Verification items for the finished model (mm, model axes). Face numbers are marked on the shaded views. A direction names the side the tool comes from. Round coordinates to 2 decimals unless told otherwise and drop trailing zeros. Loops run counter-clockwise (first coordinate to the right, second up) from the corner with the lowest first, then second, coordinate; pieces in that order, holes last. Notation, with made-up numbers: (-19.5, 33.25) -> (32.5, 33.25) arc R26 cw to (32.5, 50.25) -> close; hole circle Ø6 at (7.5, -16.5). An arc over 180 degrees is marked (long way). Use a Markdown table: item, result. Add a question column.
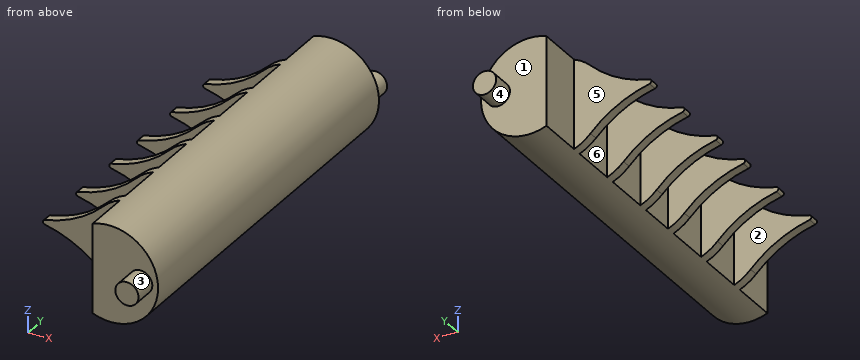
```python
from build123d import *

# Parameters (mm, degrees)
F1_DEPTH = 80
F3_DEPTH = 12.5
F4_R     = 2.5
F5_DEPTH = 5
F6_R     = 2.5
F7_DEPTH = 5


with BuildPart() as f1:
    # F0 (on Front) → F1 (new body)
    with BuildSketch(Plane.XZ):
        with BuildLine():
            ThreePointArc((9.05775, 7.130023), (3.187096, 2.771486), (-3.69351, 0.297888))
            ThreePointArc((-3.69351, 0.297888), (-4.094982, -0.192308), (-3.69351, -0.682504))
            ThreePointArc((-3.69351, -0.682504), (3.187096, -3.156101), (9.05775, -7.514638))
            ThreePointArc((9.05775, -7.514638), (26.735419, -0.192308), (9.05775, 7.130023))
        make_face()
    extrude(amount=F1_DEPTH)

    # F2 (on Top) → F3 (cut, symmetric)
    with BuildSketch(Plane.XY):
        Polygon((-6.228959, -12), (-6.228959, -10), (12.586473, -10), (12.586473, 2.989336), (-20.302792, 2.989336), (-20.302792, -84.092789), (12.586473, -84.752782), (12.586473, -70), (-6.228959, -70), (-6.228959, -68), (12.586473, -68), (12.586473, -58), (-6.228959, -58), (-6.228959, -56), (12.586473, -56), (12.586473, -46), (-5.693135, -46), (-5.693135, -44), (12.586473, -44), (12.586473, -36), (-6.228959, -36), (-6.228959, -34), (12.586473, -34), (12.586473, -24), (-6.228959, -24), (-6.228959, -22), (12.586473, -22), (12.586473, -12), align=None)
    extrude(amount=F3_DEPTH, both=True, mode=Mode.SUBTRACT)

    # F4 (on face) → F5 (join)
    with BuildSketch(Plane.XZ.offset(80)):
        with Locations((22.98077, 0)):
            Circle(F4_R)
    extrude(amount=F5_DEPTH)

    # F6 (on face) → F7 (join)
    with BuildSketch(Plane(origin=(0, 0, 0), x_dir=(-1, 0, 0), z_dir=(0, 1, 0))):
        with Locations((-22.98077, 0)):
            Circle(F6_R)
    extrude(amount=F7_DEPTH)


solid = f1.part
```
1) Release check for a two-part mould opening along Y. For the marked faces 1, 2 and 3 record: released by +Y, released by -Y, zero draft, split by the parting line, or undercut.
2) Sectioned sample at D-D on y = -47.5. Enter the section's corners in (x, z), then the cut area to 3 significant figures.
3) Sectioned sample at B-B on z = 3.5. Enter the section's corners in (x, y).
4) Access from +Z, -Z, +X, -X, +Y, -Y to the whole of each face (thin tool, end or side, straight path). Record for the marked faces 4, 5 and 6.
5) Sectioned sample at A-A on x = 7.5. Enter the section's corners in (y, z), then the cut area to 3 significant figures.
6) Thickness scan on line 1 (Y direction, x = 7, z = 1); line 2 (Y direction, x = 17.5, z = 6.5); line 3 (X direction, y = -21, z = -5.5). Record the ranges inside material, lowest first.
7) Go/stop test with flat-tipped pins: pin 1 (5 mm diameter, centred on x = 1.5, z = -0.5, fed in from +Y); pin 2 (8 mm diameter, centred on x = 1.5, z = -4.5, fed in from -Y); pin 3 (1.5 mm diameter, centred on x = 15, y = -55, fed in from +Z). Record where each tip stops, or that it passes through.
8) Sectioned sample at C-C on x = 0. Enter the section's corners in (y, z), then the cut area to 3 significant figures.
Geometry results:
| question | item | result |
|---|---|---|
| 1 | face 1 | released by +Y |
| 1 | face 2 | undercut |
| 1 | face 3 | zero draft |
| 2 | outline | (12.59, -9.83) arc R10.36 ccw (long way) to (12.59, 9.44) -> close |
| 2 | area | 245 mm^2 |
| 3 | outline | (4.46, -70) -> (12.59, -70) -> (12.59, -80) -> (26.05, -80) -> (26.05, 0) -> (12.59, 0) -> (12.59, -10) -> (4.46, -10) -> (4.46, -12) -> (12.59, -12) -> (12.59, -22) -> (4.46, -22) -> (4.46, -24) -> (12.59, -24) -> (12.59, -34) -> (4.46, -34) -> (4.46, -36) -> (12.59, -36) -> (12.59, -44) -> (4.46, -44) -> (4.46, -46) -> (12.59, -46) -> (12.59, -56) -> (4.46, -56) -> (4.46, -58) -> (12.59, -58) -> (12.59, -68) -> (4.46, -68) -> close |
| 4 | face 4 | +Y |
| 4 | face 5 | +Z, -Z, -X, +Y |
| 4 | face 6 | +Z, -Z, -X |
| 5 | outline | (-70, -6.08) -> (-68, -6.08) -> (-68, 5.7) -> (-70, 5.7) -> close; (-58, -6.08) -> (-56, -6.08) -> (-56, 5.7) -> (-58, 5.7) -> close; (-46, -6.08) -> (-44, -6.08) -> (-44, 5.7) -> (-46, 5.7) -> close; (-36, -6.08) -> (-34, -6.08) -> (-34, 5.7) -> (-36, 5.7) -> close; (-24, -6.08) -> (-22, -6.08) -> (-22, 5.7) -> (-24, 5.7) -> close; (-12, -6.08) -> (-10, -6.08) -> (-10, 5.7) -> (-12, 5.7) -> close |
| 5 | area | 141 mm^2 |
| 6 | line 1 | -70 to -68, -58 to -56, -46 to -44, -36 to -34, -24 to -22, -12 to -10 |
| 6 | line 2 | -80 to 0 |
| 6 | line 3 | 12.59 to 25.27 |
| 7 | pin 1 | y = -10 |
| 7 | pin 2 | y = -70 |
| 7 | pin 3 | z = 10.14 |
| 8 | outline | (-70, -1.73) -> (-68, -1.73) -> (-68, 1.34) -> (-70, 1.34) -> close; (-58, -1.73) -> (-56, -1.73) -> (-56, 1.34) -> (-58, 1.34) -> close; (-46, -1.73) -> (-44, -1.73) -> (-44, 1.34) -> (-46, 1.34) -> close; (-36, -1.73) -> (-34, -1.73) -> (-34, 1.34) -> (-36, 1.34) -> close; (-24, -1.73) -> (-22, -1.73) -> (-22, 1.34) -> (-24, 1.34) -> close; (-12, -1.73) -> (-10, -1.73) -> (-10, 1.34) -> (-12, 1.34) -> close |
| 8 | area | 36.8 mm^2 |
